Autodesk Inventor part; units mm, degrees
ref_plane "YZ Plane" through (0, 0, 0) normal (1, 0, 0) x (0, 1, 0)
ref_plane "XZ Plane" through (0, 0, 0) normal (0, 1, 0) x (-1, 0, 0)
ref_plane "XY Plane" through (0, 0, 0) normal (0, 0, 1) x (1, 0, 0)
sketch "Sketch1" plane through (0, 0, 0) normal (0, 0, 1) x (1, 0, 0)
  line L0 (0, 25.4) -> (-28.702, 25.4) construction
  line L1 (0, 25.4) -> (-95.25, 25.4) construction
  line L2 (-95.25, 25.4) -> (-92.075, 25.4) construction
  line L3 (-92.075, 25.4) -> (-84.455, 21.8467) construction
  line L4 (-92.075, 25.4) -> (-92.075, 22.4389) construction
  line L5 (-92.075, 0) -> (-95.25, 0)
  line L6 (-28.702, 59.0535) -> (-28.702, -92.5226) construction
  arc A0 (-28.9184, -9.8402) -> (-32.3684, -2.4417) centre (-35.052, -8.1967) ccw
  line L7 (-76.2, -186.2977) -> (-28.702, -9.0327)
  line L8 (-92.075, 25.4) -> (-92.075, 0)
  line L9 (-92.075, 25.4) -> (-32.3684, -2.4417)
  line L10 (-28.702, -8.1967) -> (-60.452, -8.1967) construction
  line L11 (-60.452, -127.5253) -> (-54.102, -127.5253) construction
  line L12 (-54.102, -127.5253) -> (-54.102, -103.8268) construction
  line L13 (-54.102, -103.8268) -> (-60.452, -103.8268)
  line L14 (-60.452, 10.654) -> (-60.452, 1.129) construction
  line L15 (-60.452, 10.654) -> (-60.452, 4.1232) construction
  line L16 (-60.452, 4.1232) -> (-46.4468, 4.1232)
  line L17 (-95.25, 0) -> (-95.25, -12.7) construction
  line L18 (-60.452, -12.7) -> (-73.152, -12.7) construction
  line L19 (-95.25, -12.7) -> (-95.25, -25.4) construction
  line L20 (-95.25, -25.4) -> (-95.25, -88.9) construction
  line L21 (-95.25, -88.9) -> (-82.55, -88.9) construction
  line L22 (-82.55, -88.9) -> (-82.55, -25.4) construction
  line L23 (-95.25, -25.4) -> (-82.55, -25.4)
  line L24 (-82.55, -25.4) -> (-82.55, -88.9)
  line L25 (-82.55, -88.9) -> (-95.25, -88.9)
  line L26 (-95.25, -12.7) -> (-73.152, -12.7)
  line L27 (-73.152, -139.3746) -> (-63.627, -139.3746)
  line L28 (-82.55, -88.9) -> (-82.55, -186.2977)
  line L29 (-82.55, -186.2977) -> (-76.2, -186.2977)
  line L30 (-73.152, -12.7) -> (-73.152, -139.3746)
  line L31 (-88.9, -25.4) -> (-88.9, -31.3436)
  line L32 (-88.9, -31.3436) -> (-95.25, -31.3436)
  line L33 (-95.25, 0) -> (-95.25, -25.4)
  line L34 (-95.25, -31.3436) -> (-95.25, -88.9)
  line L35 (-88.9, -160.8977) -> (-88.9, -221.8454)
  line L36 (-28.9184, -9.8402) -> (-85.725, -221.8454)
  line L37 (-85.725, -221.8454) -> (-88.9, -221.8454)
  line L38 (-82.55, -160.8977) -> (-88.9, -160.8977)
  line L39 (-66.802, -38.1) -> (-66.802, 4.1232)
  line L40 (-66.802, 4.1232) -> (-60.452, 4.1232)
  line L41 (-66.802, -38.1) -> (-60.452, -103.8268)
  line L42 (-60.452, 10.654) -> (-60.452, 4.1232) construction
  line L43 (-60.452, -8.1967) -> (-60.452, -12.7) construction
  line L44 (-60.452, -103.8268) -> (-60.452, -127.5253) construction
  line L45 (0, 59.6457) -> (0, -91.9304) construction
  line L46 (-73.152, -38.1) -> (-69.977, -38.1)
  line L47 (-69.977, -38.1) -> (-69.977, -12.7)
  line L48 (-66.802, -12.7) -> (-69.977, -12.7)
  point P0 (0, 0)
  point P1 (-95.25, -256.5049)
  point P2 (-88.7095, 22.4389)
  dimension "d0" = 28.702
  dimension "d1" = 95.25
  dimension "d2" = 3.175
  dimension "d3" = 25
  dimension "d5" = 25.4
  dimension "d6" = 25.4
  dimension "d8" = 12.7
  dimension "d12" = 31.75
  dimension "d13" = 6.35
  dimension "d16" = 12.7
  dimension "d17" = 12.7
  dimension "d18" = 12.7
  dimension "d19" = 63.5
  dimension "d20" = 12.7
  dimension "d22" = 9.525
  dimension "d23" = 6.35
  dimension "d25" = 5.9436
  dimension "d27" = 3.175
  dimension "d28" = 6.35
  dimension "d29" = 25.4
  dimension "d30" = 107.95
  dimension "d31" = 6.35
  dimension "d33" = 20.3552
  dimension "d34" = 15
  dimension "d35" = 3.175
  dimension "d36" = 25.4
revolve "Revolution2" add sketch "Sketch1" angle 360 about axis through (0, 59.6457, 0) along (0, -1, 0) contours L9 A0 L7 L13 L41 L39 L40 L16
properties part number "graphite" material "Graphite"
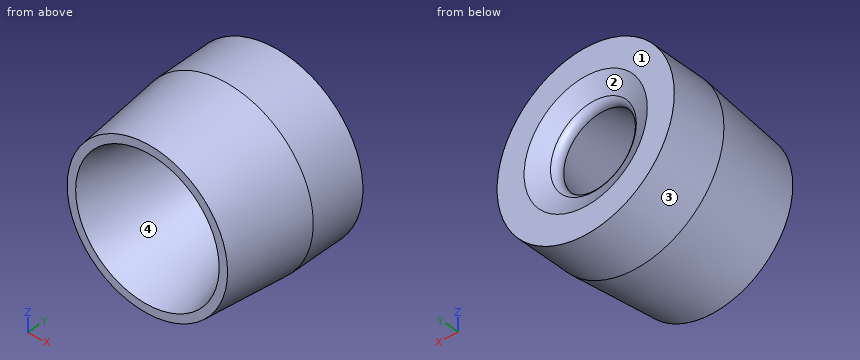
Here's how the part is built. I have some questions about the finished solid (model axes, mm). Face numbers are marked on the shaded views. Round coordinates to 2 decimals unless told otherwise and drop trailing zeros. Write each loop counter-clockwise with the first axis right and the second up, starting at its lowest first coordinate (ties: lowest second). Pieces come first, ordered by that corner, then holes.
Q1. If we section it at A-A on x = 0: Write out the boundary of the cut face in (y, z), plus the area to 3 significant figures.
Q2. Please list where these lines run through material, in increasing order: probe 1 along Z at (x, y) = (20.5, -48); probe 2 along X at (y, z) = (-68, 21); probe 3 along Z at (x, y) = (5, -50).
Q3. Will these pins go through, and if not, where does the flat tip stop? P1, Ø10, axis at x = 7, y = -33, coming from the +Z side; P2, Ø3, axis at x = -10, z = 28, coming from the +Y side; P3, Ø1.5, axis at y = -82, z = -49.5, coming from the +X side.
Q4. If we section it at C-C on y = -13: Write out the boundary of the cut face in (x, z).
Q5. If we section it at D-D on y = -85: Write out the boundary of the cut face in (x, z), plus the area to 3 significant figures.
Q6. If we mould it in two halves opening along X, with no side actions, what happens to the marked faces 1, 2, 3 and 4? For each: +X half, -X half, draft (parallel to the pull), parting line (faces both ways), or undercut.
Q7. If we section it at B-B on z = 0: Write out the boundary of the cut face in (x, y).
Answer below:
1. outline: (-103.83, -60.45) - (-38.1, -66.8) - (4.12, -66.8) - (4.12, -46.45) - (-2.44, -32.37) arc R6.35 ccw to (-9.84, -28.92) - (-103.83, -54.1) - close; (-103.83, 54.1) - (-9.84, 28.92) arc R6.35 ccw to (-2.44, 32.37) - (4.12, 46.45) - (4.12, 66.8) - (-38.1, 66.8) - (-103.83, 60.45) - close
1. area: 5,250 mm2
2. probe 1: z = -62.57 to -33.35, 33.35 to 62.57
2. probe 2: x = -60.36 to -39.24, 39.24 to 60.36
2. probe 3: z = -65.46 to -39.36, 39.36 to 65.46
3. P1: stops at z = 66.77
3. P2: stops at y = -3.12
3. P3: stops at x = 39.22
4. outline: circle Ø133.6 at (0, 0); hole circle Ø59.53 at (0, 0)
5. outline: circle Ø124.54 at (0, 0); hole circle Ø98.11 at (0, 0)
5. area: 4,620 mm2
6. face 1: draft
6. face 2: undercut
6. face 3: parting line
6. face 4: undercut
7. outline: (-66.8, -38.1) - (-60.45, -103.83) - (-54.1, -103.83) - (-28.92, -9.84) arc R6.35 ccw to (-32.37, -2.44) - (-46.45, 4.12) - (-66.8, 4.12) - close; (28.92, -9.84) - (54.1, -103.83) - (60.45, -103.83) - (66.8, -38.1) - (66.8, 4.12) - (46.45, 4.12) - (32.37, -2.44) arc R6.35 ccw to start
